Input: part model. Units: mm. Frame: model coordinates. A direction names the side the tool comes from. Round coordinates to 2 decimals unless told otherwise and drop trailing zeros. Order: outer loops, then holes, each group sorted by start corner. A loop starts at its lowest first (then second) coordinate and runs counter-clockwise, first axis right, second up.
Item 1: Cut plane B-B on z = -8.5. Output: boundary loops of the cut face in (x, y), then the cut area to 3 significant figures.
Item 2: Cut plane A-A on y = -13.5. Output: boundary loops of the cut face in (x, z).
Item 3: Cut plane C-C on x = -57. Output: boundary loops of the cut face in (y, z).
Item 4: Line query: L1, parallel to X at y = 4.5, z = 17.5; L2, parallel to Z at x = -26.5, y = -10.5; L3, parallel to Z at x = -68, y = 5.5. Output: solid intervals per line, ascending.
Item 5: First-contact query: pin 1 (5 mm diameter, centred on x = -61.5, z = 2, fed in from +Y); pin 2 (6 mm diameter, centred on x = -45, y = -14, fed in from +Z); pin 3 (22 mm diameter, centred on x = -69.5, y = -4.5, fed in from -Z); pin 4 (25 mm diameter, centred on y = 10, z = -12, fed in from -X). Flat tips, straight axial feed; report the tip coordinate or a pass-through.
Item 6: Reachability of faces 1 (the flat face through (-40, 0, 15.613)), 2 (the flat face through (-65, -10, 0)), 3 (the flat face through (-65, 0, -10)), 4 (the flat face through (-65, 10, 0)) from +Z, -Z, +X, -X, +Y, -Y: full face, straight path, thin tool, end or side. Return the list, or none.
Item 7: Cut plane D-D on y = 5. Output: boundary loops of the cut face in (x, z).
```python
from build123d import *

# Parameters (mm, degrees)
F0_W     = 50
F0_H     = 50
F1_DEPTH = 25
F2_W     = 30
F2_H     = 30
F3_DEPTH = 30
F4_W     = 20
F4_H     = 20
F5_DEPTH = 20


with BuildPart() as f1:
    # F0 (on Front) → F1 (new body, symmetric)
    with BuildSketch(Plane.XZ):
        Rectangle(F0_W, F0_H)
    extrude(amount=F1_DEPTH, both=True)

    # F2 (on face) → F3 (join)
    with BuildSketch(Plane(origin=(-25, 0, 0), x_dir=(0, -1, 0), z_dir=(-1, 0, 0))):
        with Locations((0, 0.612991)):
            Rectangle(F2_W, F2_H)
    extrude(amount=F3_DEPTH)

    # F4 (on face) → F5 (join)
    with BuildSketch(Plane(origin=(-55, 0, 0), x_dir=(0, -1, 0), z_dir=(-1, 0, 0))):
        Rectangle(F4_W, F4_H)
    extrude(amount=F5_DEPTH)


solid = f1.part
```
From the geometry:
1. outline: (-75, -10) - (-55, -10) - (-55, -15) - (-25, -15) - (-25, -25) - (25, -25) - (25, 25) - (-25, 25) - (-25, 15) - (-55, 15) - (-55, 10) - (-75, 10) - close
1. area: 3,800 mm2
2. outline: (-55, -14.39) - (-25, -14.39) - (-25, -25) - (25, -25) - (25, 25) - (-25, 25) - (-25, 15.61) - (-55, 15.61) - close
3. outline: (-10, -10) - (10, -10) - (10, 10) - (-10, 10) - close
4. L1: x = -25 to 25
4. L2: z = -14.39 to 15.61
4. L3: z = -10 to 10
5. pin 1: stops at y = 10
5. pin 2: stops at z = 15.61
5. pin 3: stops at z = -10
5. pin 4: stops at x = -75
6. face 1: +Z, -X, +Y, -Y
6. face 2: +Z, -Z, -X, -Y
6. face 3: -Z, -X, +Y, -Y
6. face 4: +Z, -Z, -X, +Y
7. outline: (-75, -10) - (-55, -10) - (-55, -14.39) - (-25, -14.39) - (-25, -25) - (25, -25) - (25, 25) - (-25, 25) - (-25, 15.61) - (-55, 15.61) - (-55, 10) - (-75, 10) - close
